CAD build for the part. Positions are in the model's coordinates, mm. Face numbers are marked on the shaded views. A direction names the side the tool comes from. Coordinates: 2 decimals unless noted, no trailing zeros. Loops run counter-clockwise (first coordinate to the right, second up) from the corner with the lowest first, then second, coordinate; pieces in that order, holes last.
1) Pin check, flat tips, straight feed: pin 1 Ø1.5 at (x, z) = (-57.5, 2) entering from +Y; pin 2 Ø2 at (x, y) = (-47.79, 88.4) entering from +Z; pin 3 Ø1 at (y, z) = (87, 4.5) entering from -X; pin 4 Ø2 at (x, y) = (-47.5, 89.5) entering from -Z. Stop position of each tip, or through.
2) Saw through at A-A, the plane z = 2. Write the cut outline in (x, y), and give its area (3 significant figures).
3) Which spindle directions (+Z, -Z, +X, -X, +Y, -Y) get a long thin tool onto all of the face, cutting with end or side? Do the marked faces 1, 2, 3, 4 and 5. Say none if no direction does.
4) Saw through at D-D, the plane z = 4.25. Write the cut outline in (x, y), and give its area (3 significant figures).
5) Wall check: line 1 along X through (y, z) = (85.75, 1); line 2 along Z through (x, y) = (-49, 86.25); line 3 along Z through (x, y) = (-43.75, 85). Give the ranges that are in metal, low to high.
6) Two-plate mould, pull along X, no slides. Class the marked faces 6, 7 and 8: +X half, -X half, draft (parallel to the pull), parting line (faces both ways), or undercut.
7) Saw through at B-B, the plane x = -39.5. Write the cut outline in (y, z), and give its area (3 significant figures).
8) Saw through at C-C, the plane y = 92. Write the cut outline in (x, z).
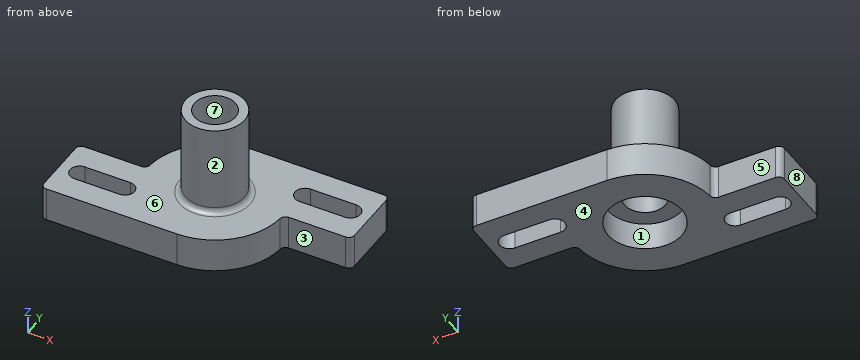
```python
from build123d import *

# Parameters (mm, degrees)
BOSS_EXTRUDE1_DEPTH                                  = 3
SKETCH2_R                                            = 2.6
BOSS_EXTRUDE2_DEPTH                                  = 8
FILLET1_R                                            = 0.5
CBORE_FOR_M3_HEX_SOCKET_THIN_HEAD_CAP_SC_D           = 3.6
CBORE_FOR_M3_HEX_SOCKET_THIN_HEAD_CAP_SC_CBORE_D     = 6.5
CBORE_FOR_M3_HEX_SOCKET_THIN_HEAD_CAP_SC_CBORE_DEPTH = 2.4


with BuildPart() as part:
    # Sketch1 → Boss-Extrude1 (new body)
    with BuildSketch(Plane.XY):
        with BuildLine():
            Line((-47.789798407, 94.395653496), (-35.789798407, 94.395653496))
            Line((-35.789798407, 94.395653496), (-35.789798407, 88.395653496))
            Line((-35.789798407, 88.395653496), (-41.789798407, 88.395653496))
            ThreePointArc((-41.789798407, 88.395653496), (-43.54715772, 84.153012809), (-47.789798407, 82.395653496))
            Line((-47.789798407, 82.395653496), (-59.789798407, 82.395653496))
            Line((-59.789798407, 82.395653496), (-59.789798407, 88.395653496))
            Line((-59.789798407, 88.395653496), (-53.789798407, 88.395653496))
            ThreePointArc((-53.789798407, 88.395653496), (-52.032439094, 92.638294183), (-47.789798407, 94.395653496))
        make_face()
        with BuildLine():
            Line((-37.539798407, 90.516657199), (-41.539798407, 90.516657199))
            ThreePointArc((-41.539798407, 90.516657199), (-42.418794704, 91.395653496), (-41.539798407, 92.274649793))
            Line((-41.539798407, 92.274649793), (-37.539798407, 92.274649793))
            ThreePointArc((-37.539798407, 92.274649793), (-36.66080211, 91.395653496), (-37.539798407, 90.516657199))
        make_face(mode=Mode.SUBTRACT)
        with BuildLine():
            Line((-58.039798407, 86.229692735), (-54.039798407, 86.229692735))
            ThreePointArc((-54.039798407, 86.229692735), (-53.205759169, 85.395653496), (-54.039798407, 84.561614258))
            Line((-54.039798407, 84.561614258), (-58.039798407, 84.561614258))
            ThreePointArc((-58.039798407, 84.561614258), (-58.873837646, 85.395653496), (-58.039798407, 86.229692735))
        make_face(mode=Mode.SUBTRACT)
    extrude(amount=BOSS_EXTRUDE1_DEPTH)

    # Sketch2 → Boss-Extrude2 (add)
    with BuildSketch(Plane(origin=(0, 0, 3), x_dir=(-1, 0, 0), z_dir=(0, 0, -1))):
        with Locations((47.789798407, 88.395653496)):
            Circle(SKETCH2_R)
    extrude(amount=-BOSS_EXTRUDE2_DEPTH)

    # Fillet1
    fillet1_edges = [part.edges().sort_by_distance(p)[0] for p in [
        (-35.789798407, 94.395653496, 1.5),
        (-35.789798407, 88.395653496, 1.5),
        (-41.789798407, 88.395653496, 1.5),
        (-59.789798407, 82.395653496, 1.5),
        (-59.789798407, 88.395653496, 1.5),
        (-53.789798407, 88.395653496, 1.5),
        (-45.189798407, 88.395653496, 3),
    ]]
    fillet(fillet1_edges, radius=FILLET1_R)

    # CBORE for M3 Hex Socket Thin Head Cap Screw1 (through all)
    with Locations(Plane(origin=(0, 0, 0), x_dir=(-1, 0, 0), z_dir=(0, 0, -1))):
        with Locations((47.789798407, 88.395653496)):
            CounterBoreHole(CBORE_FOR_M3_HEX_SOCKET_THIN_HEAD_CAP_SC_D / 2, CBORE_FOR_M3_HEX_SOCKET_THIN_HEAD_CAP_SC_CBORE_D / 2, CBORE_FOR_M3_HEX_SOCKET_THIN_HEAD_CAP_SC_CBORE_DEPTH)


solid = part.part
```
Data:
1. pin 1: stops at y = 88.4
1. pin 2: passes through
1. pin 3: stops at x = -50.23
1. pin 4: stops at z = 2.4
2. outline: (-59.79, 82.9) arc R0.5 ccw to (-59.29, 82.4) - (-47.79, 82.4) arc R6 ccw to (-41.81, 87.93) arc R0.5 cw to (-41.31, 88.4) - (-36.29, 88.4) arc R0.5 ccw to (-35.79, 88.9) - (-35.79, 93.9) arc R0.5 ccw to (-36.29, 94.4) - (-47.79, 94.4) arc R6 ccw to (-53.77, 88.86) arc R0.5 cw to (-54.27, 88.4) - (-59.29, 88.4) arc R0.5 ccw to (-59.79, 87.9) - close; hole (-58.04, 84.56) - (-54.04, 84.56) arc R0.83 ccw to (-54.04, 86.23) - (-58.04, 86.23) arc R0.83 ccw to start; hole circle Ø6.5 at (-47.79, 88.4); hole (-41.54, 90.52) - (-37.54, 90.52) arc R0.88 ccw to (-37.54, 92.27) - (-41.54, 92.27) arc R0.88 ccw to start
2. area: 149 mm2
3. face 1: -Z
3. face 2: +Z
3. face 3: +Z, -Z, +X, -Y
3. face 4: -Z, +X, -X, +Y, -Y
3. face 5: +Z, -Z, -X, +Y
4. outline: circle Ø5.2 at (-47.79, 88.4); hole circle Ø3.6 at (-47.79, 88.4)
4. area: 11.1 mm2
5. line 1: x = -59.79 to -58.79, -53.28 to -49.68, -45.9 to -42.4
5. line 2: z = 2.4 to 11
5. line 3: z = 0 to 3
6. face 6: draft
6. face 7: undercut
6. face 8: -X half
7. outline: (88.4, 0) - (90.52, 0) - (90.52, 3) - (88.4, 3) - close; (92.27, 0) - (94.4, 0) - (94.4, 3) - (92.27, 3) - close
7. area: 12.7 mm2
8. outline: (-52.59, 0) - (-42.18, 0) - (-42.18, 3) - (-52.59, 3) - close; (-36.9, 0) - (-35.79, 0) - (-35.79, 3) - (-36.9, 3) - close
